The listing builds one solid part. Answer for the finished solid, in the listing's coordinates (mm). Face numbers are marked on the shaded views. A direction names the side the tool comes from. Give positions to 0.01 mm unless a question says otherwise; leave off trailing zeros. Order: outer loops, then holes, each group sorted by start corner. A loop starts at its lowest first (then second) coordinate and runs counter-clockwise, first axis right, second up. Notation, with made-up numbers: (88, 69.25) -> (96, 69.25) arc R12 cw to (96, 79.25) -> close; hole circle Ø4 at (70, 21.5). An arc over 180 degrees is marked (long way). One line per question, with ' | ' between items. Start each with the question number.
```python
from build123d import *

# Parameters (mm, degrees)
F0_R      = 50.675
F1_DEPTH  = 95.25
F6_R      = 64.2548627896
F7_DEPTH  = 63.5
F10_DEPTH = 31.751


# Not quite as in the source:
# - a feature of the source that left no trace in its solid (it failed there, or was rolled back) is left out


with BuildPart() as f1:
    # F0 (on Top) → F1 (new body)
    with BuildSketch(Plane.XY):
        Circle(F0_R)
    extrude(amount=F1_DEPTH)

    # F2 (on Front) → F3 (revolve, cut)
    with BuildSketch(Plane.XZ):
        Polygon((-50.6984, 0), (-31.75, 0), (-50.6984, 12.7), align=None)
    revolve(axis=Axis((0, 0, 21.0587424167), (0, 0, 1)), mode=Mode.SUBTRACT)

    # F4 (on Front) → F5 (revolve, cut)
    with BuildSketch(Plane.XZ):
        Polygon((0, 0.6), (0, 108.2893535495), (-15, 108.2893535495), (-15, 17.6), (-3.5, 0.6), align=None)
    revolve(axis=Axis((0, 0, 54.4446767747), (0, 0, -1)), mode=Mode.SUBTRACT)

    # F6 (on face) → F7 (cut)
    with BuildSketch(Plane.XY.offset(95.25)):
        Circle(F6_R)
    extrude(amount=-F7_DEPTH, mode=Mode.SUBTRACT)

    # F9 (on face) → F10 (cut, through all)
    with BuildSketch(Plane.XY.offset(31.75)):
        with BuildLine():
            ThreePointArc((-11.7065258502, 25.1047257009), (0, 27.7), (11.7065258502, 25.1047257009))
            Line((11.7065258502, 25.1047257009), (19.2692796441, 41.3231035499))
            ThreePointArc((19.2692796441, 41.3231035499), (0, 45.595), (-19.2692796441, 41.3231035499))
            Line((-19.2692796441, 41.3231035499), (-11.7065258502, 25.1047257009))
        make_face()
        with BuildLine():
            ThreePointArc((-27.4935284005, -3.3757808123), (-26.3442655014, 8.5597707442), (-20.2584975349, 18.8913545737))
            Line((-20.2584975349, 18.8913545737), (-33.3460720253, 31.095715227))
            ThreePointArc((-33.3460720253, 31.095715227), (-43.3634218605, 14.0896298585), (-45.2551417841, -5.5566327126))
            Line((-45.2551417841, -5.5566327126), (-27.4935284005, -3.3757808123))
        make_face()
        with BuildLine():
            ThreePointArc((-5.2854091719, -27.1910729815), (-16.2816514885, -22.4097707442), (-24.2269658878, -13.4292264808))
            Line((-24.2269658878, -13.4292264808), (-39.878285547, -22.1048946351))
            ThreePointArc((-39.878285547, -22.1048946351), (-26.8000685783, -36.8871298585), (-8.6999361442, -44.7572914293))
            Line((-8.6999361442, -44.7572914293), (-5.2854091719, -27.1910729815))
        make_face()
        with BuildLine():
            ThreePointArc((24.2269658878, -13.4292264808), (16.2816514885, -22.4097707442), (5.2854091719, -27.1910729815))
            Line((5.2854091719, -27.1910729815), (8.6999361442, -44.7572914293))
            ThreePointArc((8.6999361442, -44.7572914293), (26.8000685783, -36.8871298585), (39.878285547, -22.1048946351))
            Line((39.878285547, -22.1048946351), (24.2269658878, -13.4292264808))
        make_face()
        with BuildLine():
            ThreePointArc((20.2584975349, 18.8913545737), (26.3442655014, 8.5597707442), (27.4935284005, -3.3757808123))
            Line((27.4935284005, -3.3757808123), (45.2551417841, -5.5566327126))
            ThreePointArc((45.2551417841, -5.5566327126), (43.3634218605, 14.0896298585), (33.3460720253, 31.095715227))
            Line((33.3460720253, 31.095715227), (20.2584975349, 18.8913545737))
        make_face()
    extrude(amount=-F10_DEPTH, mode=Mode.SUBTRACT)


solid = f1.part
```
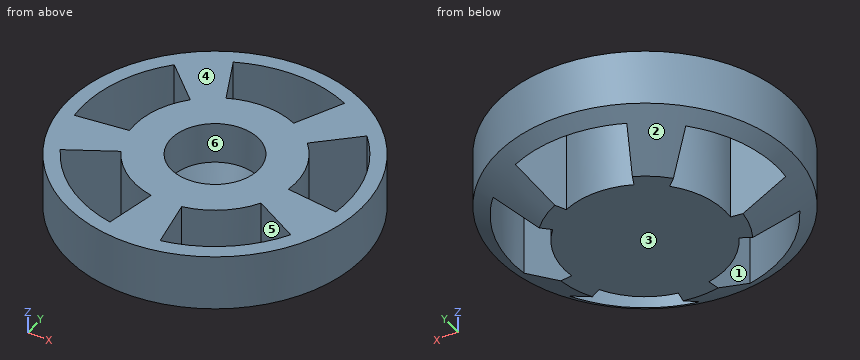
(1) The part is cut by section D-D on z = 2.5. Determine the outline of the cut face in (x, y).
(2) Given P1, Ø3, axis at y = 37.5, z = 13, coming from the -X side; P2, Ø12, axis at x = 37, z = 22.5, coming from the -Y side; P3, Ø3, axis at y = 2, z = 6, coming from the -X side; P4, Ø6, axis at x = -40, y = -37.5, coming from the -Z side, each flat-ended and moving along its own axis, determine where each tip first touches the part or whether it passes through.
(3) Consider line 1 (X direction, y = 4, z = 25.5); line 2 (X direction, y = -34, z = 16); line 3 (X direction, y = -24, z = 14.5). Determine where each line is inside the solid, lowest interval first.
(4) Determine the mould class of the marked faces 1, 2 and 3 for opening direction X: pulls with the +X half, pulls with the -X half, needs draft (parallel to the pull), parting line crosses it, or undercut.
(5) For the marked faces 4, 5 and 6, determine the directions among +Z, -Z, +X, -X, +Y, -Y from which every point of the face is accessible in a straight line to the end or side of a thin tool.
(6) The part is cut by section A-A on z = 20. State how many separate pieces and enclosed holes the cut face has, plus the area to 3 significant figures.
Result sheet:
1) outline: (-35.22, -4.32) arc R35.48 ccw to (-31.03, -17.2) -> (-24.23, -13.43) arc R27.7 ccw to (-5.29, -27.19) -> (-6.77, -34.83) arc R35.48 ccw to (6.77, -34.83) -> (5.29, -27.19) arc R27.7 ccw to (24.23, -13.43) -> (31.03, -17.2) arc R35.48 ccw to (35.22, -4.32) -> (27.49, -3.38) arc R27.7 ccw to (20.26, 18.89) -> (25.95, 24.2) arc R35.48 ccw to (14.99, 32.16) -> (11.71, 25.1) arc R27.7 ccw to (-11.71, 25.1) -> (-14.99, 32.16) arc R35.48 ccw to (-25.95, 24.2) -> (-20.26, 18.89) arc R27.7 ccw to (-27.49, -3.38) -> close; hole circle Ø9.57 at (0, 0)
2) P1: stops at x = -35.66 | P2: stops at y = -40.09 | P3: stops at x = -27.7 | P4: passes through
3) line 1: x = -50.52 to -45.42, -27.41 to -14.46, 14.46 to 27.41, 45.42 to 50.52 | line 2: x = -37.58 to -30.38, -6.61 to 6.61, 30.38 to 37.58 | line 3: x = -44.63 to -38.77, -13.83 to 13.83, 38.77 to 44.63
4) face 1: undercut | face 2: parting line crosses it | face 3: needs draft
5) face 4: +Z, +X, -X, +Y, -Y | face 5: +Z, -Z | face 6: +Z
6) separate pieces: 1 | enclosed holes: 6 | area: 4,500 mm^2
